```python
from build123d import *

# Parameters (mm, degrees)
BOSS_EXTRU_1_DEPTH      = 3
ESQUISSE2_W             = 5
ESQUISSE2_H             = 4
ENL_V_MAT_EXTRU_1_DEPTH = 3
ESQUISSE4_R             = 1.8
ENL_V_MAT_EXTRU_2_DEPTH = 3
ENL_V_MAT_EXTRU_3_DEPTH = 3


with BuildPart() as part:
    # Esquisse1 → Boss.-Extru.1 (new body)
    with BuildSketch(Plane.XY):
        Polygon((-220, 50), (-40, -110), (40, -110), (220, 50), (220, 110), (-220, 110), align=None)
    extrude(amount=BOSS_EXTRU_1_DEPTH)

    # Esquisse2 → Enlèv. mat.-Extru.1 (cut)
    with BuildSketch(Plane(origin=(0, 0, 0), x_dir=(-1, 0, 0), z_dir=(0, 0, -1))):
        with Locations((-201.5, 95)):
            Rectangle(ESQUISSE2_W, ESQUISSE2_H)
        with Locations((-168.5, 95)):
            Rectangle(ESQUISSE2_W, ESQUISSE2_H)
        with Locations((-168.5, 61)):
            Rectangle(ESQUISSE2_W, ESQUISSE2_H)
        with Locations((-201.5, 61)):
            Rectangle(ESQUISSE2_W, ESQUISSE2_H)
        with Locations((168.5, 61)):
            Rectangle(ESQUISSE2_W, ESQUISSE2_H)
        with Locations((201.5, 61)):
            Rectangle(ESQUISSE2_W, ESQUISSE2_H)
        with Locations((168.5, 95)):
            Rectangle(ESQUISSE2_W, ESQUISSE2_H)
        with Locations((201.5, 95)):
            Rectangle(ESQUISSE2_W, ESQUISSE2_H)
        with Locations((-16.5, -48)):
            Rectangle(ESQUISSE2_W, ESQUISSE2_H)
        with Locations((16.5, -48)):
            Rectangle(ESQUISSE2_W, ESQUISSE2_H)
        with Locations((16.5, -82)):
            Rectangle(ESQUISSE2_W, ESQUISSE2_H)
        with Locations((-16.5, -82)):
            Rectangle(ESQUISSE2_W, ESQUISSE2_H)
    extrude(amount=-ENL_V_MAT_EXTRU_1_DEPTH, mode=Mode.SUBTRACT)

    # Esquisse4 → Enlèv. mat.-Extru.2 (cut)
    with BuildSketch(Plane.XY.offset(3)):
        with Locations((-37, 50)):
            Circle(ESQUISSE4_R)
        with Locations((37, 50)):
            Circle(ESQUISSE4_R)
        with Locations((-37, -10)):
            Circle(ESQUISSE4_R)
        with Locations((37, -10)):
            Circle(ESQUISSE4_R)
    extrude(amount=-ENL_V_MAT_EXTRU_2_DEPTH, mode=Mode.SUBTRACT)

    # Esquisse5 → Enlèv. mat.-Extru.3 (cut)
    with BuildSketch(Plane.XY.offset(3)):
        Polygon((-145, 90), (-60, 90), (-60, -65), (-145, 10.555555556), align=None)
        Polygon((145, 90), (60, 90), (60, -65), (145, 10.555555556), align=None)
    extrude(amount=-ENL_V_MAT_EXTRU_3_DEPTH, mode=Mode.SUBTRACT)


solid = part.part
```
Verification items for the finished model (mm, model axes). A direction names the side the tool comes from. Coordinates: 2 decimals unless noted, no trailing zeros. Loops run counter-clockwise (first coordinate to the right, second up) from the corner with the lowest first, then second, coordinate; pieces in that order, holes last. Notation, with made-up numbers: (-15.5, 50) - (26.5, 50) arc R26 ccw to (26.5, 74) - close; hole circle Ø8 at (53.5, 78). An arc over 180 degrees is marked (long way). Return JSON: item names as keys, results as strings.
1. Section check A-A, the plane y = 81. Record the boundary of the cut face in (x, z).
Established:
{"outline": "(-220, 0) - (-145, 0) - (-145, 3) - (-220, 3) - close; (-60, 0) - (60, 0) - (60, 3) - (-60, 3) - close; (145, 0) - (220, 0) - (220, 3) - (145, 3) - close"}
2. Mould release check, pull along X, two halves, no side actions. Record for faces 3 (the flat face through (128.74, -31.12, 1.48)), 4 (the flat face through (-3, 26, 3)), 5 (the flat face through (-101.905, -27.751, 1.521)): +X half, -X half, draft (parallel to the pull), parting line (faces both ways), or undercut.
Established:
{"face 3": "+X half", "face 4": "draft", "face 5": "undercut"}
3. Section check D-D, the plane x = 153. Record the boundary of the cut face in (y, z), then the cut area to 3 significant figures.
Established:
{"outline": "(-9.56, 0) - (110, 0) - (110, 3) - (-9.56, 3) - close", "area": "359 mm2"}
4. Section check C-C, the plane z = 1.3. Count the separate pieces of the cut face and the enclosed holes in it, then the cut area to 3 significant figures.
Established:
{"separate pieces": "1", "enclosed holes": "18", "area": "47,800 mm2"}
5. Section check B-B, the plane y = 26. Record the boundary of the cut face in (x, z).
Established:
{"outline": "(-193, 0) - (-145, 0) - (-145, 3) - (-193, 3) - close; (-60, 0) - (60, 0) - (60, 3) - (-60, 3) - close; (145, 0) - (193, 0) - (193, 3) - (145, 3) - close"}
6. Thickness scan on L1, parallel to X at y = 95.5, z = 1.55; L2, parallel to Y at x = 37, z = 1.1; L3, parallel to X at y = 66.5, z = 1.6. Record the ranges inside material, lowest first.
Established:
{"L1": "x = -220 to -204, -199 to -171, -166 to 166, 171 to 199, 204 to 220", "L2": "y = -110 to -11.8, -8.2 to 48.2, 51.8 to 110", "L3": "x = -220 to -145, -60 to 60, 145 to 220"}
7. Go/stop test with flat-tipped pins: pin 1 (1.5 mm diameter, centred on x = -69, z = 1, fed in from -Y); pin 2 (1.5 mm diameter, centred on x = -168, z = 1, fed in from -Y); pin 3 (0.9 mm diameter, centred on y = -82, z = 1.5, fed in from -X). Record where each tip stops, or that it passes through.
Established:
{"pin 1": "stops at y = -84.89", "pin 2": "stops at y = 3.11", "pin 3": "stops at x = -72.01"}
8. Tool access check on faces 1 (the flat face through (101.905, -27.751, 1.521)), 2 (the flat face through (-3, 26, 0)). Record the directions out of +Z, -Z, +X, -X, +Y, -Y that give a thin tool (end or side, any length) a straight path to the whole face; none if there is none.
Established:
{"face 1": "+Z, -Z", "face 2": "-Z, +X, -X, +Y, -Y"}
